Work out the finished part from the listing and answer in its coordinate system (mm). A direction names the side the tool comes from. Give positions to 0.01 mm unless a question says otherwise; leave off trailing zeros. Order: outer loops, then holes, each group sorted by start corner. A loop starts at its lowest first (then second) coordinate and runs counter-clockwise, first axis right, second up.
```python
from build123d import *

# Parameters (mm, degrees)
F0_R            = 125
F1_DEPTH        = 1000
F6_DEPTH        = 25
F6_COPIES_COUNT = 6


# Not quite as in the source:
# - a fillet or chamfer that OpenCascade refuses, or shapes differently, is made with other operations: its cross-section is extruded or revolved along the edge and cut away or added
# - a pattern or mirror of a feature is missing from the dataset's text; its kind, count and spacing are read off the source's solid


with BuildPart() as f1:
    # F0 (on Top) → F1 (new body)
    with BuildSketch(Plane.XY):
        Circle(F0_R)
    extrude(amount=F1_DEPTH)

    # F2 (on Front) → F3 (revolve)
    with BuildSketch(Plane.XZ):
        Polygon((-124.5536804199, 997.6518154144), (0, 998.6120462418), (0, 1213.404417038), align=None)
    revolve(axis=Axis((0, 0, 1106.0082316399), (0, 0, 1)))

    # F4: fillet of radius 5 on 1 edges, made by hand

    # F4_s1 → F4_t2 (revolve, cut)
    with BuildSketch(Plane.XZ):
        with BuildLine():
            ThreePointArc((125, 996.1565242927), (124.5271615516, 998.2789776575), (123.1980766857, 1000))
            Line((123.1980766857, 1000), (125, 1000))
            Line((125, 1000), (125, 996.1565242927))
        make_face()
    revolve(axis=Axis((0, 0, 1000), (0, 0, 1)), mode=Mode.SUBTRACT)

    # F5 (on Front) → F6 (join)
    with BuildSketch(Plane.XZ):
        Polygon((0, 300), (0, 0), (250, 0), align=None)
    f6 = extrude(amount=F6_DEPTH)

    # F6_copies: F6 ×6 about axis
    f6_copies_axis = Axis((0, 0, 0), (0, 0, 1))
    for i in range(1, F6_COPIES_COUNT):
        add(f6.rotate(f6_copies_axis, i * 360 / F6_COPIES_COUNT))


solid = f1.part
```
1. Which of the six approach directions +Z, -Z, +X, -X, +Y, -Y give full straight-line access (tool end or side, diameter ignored) to faces 1 (the face through (56.85, -148.47, 43.58)), 2 (the face through (79.424, -137.566, 42.717)), 3 (the face through (-56.85, 148.47, 43.58)), 4 (the face through (-100.153, -123.471, 43.58)), 5 (the face through (-124.88, 5.5, 491.11))?
Findings below:
face 1: +Z, -Z, -Y
face 2: +Z, -Z, +X
face 3: +Z, -Z, +Y
face 4: +Z, -Z, -X
face 5: +Z
2. The part is cut by section C-C (x = 207.5). Write down the section's boundary in (y, z), then the cut area to 4 significant figures.
Findings below:
outline: (-25, 0) - (0, 0) - (0, 51) - (-25, 51) - close
area: 1,275 mm2
3. The mould has two halves that part along X. Classify faces 6 (the face through (-79.424, -137.566, 42.717)), 7 (the face through (187.13, -12.325, 75.444)), 8 (the face through (-104.24, -155.9, 75.44)): pulls with the +X half, pulls with the -X half, needs draft (parallel to the pull), parting line crosses it, or undercut.
Findings below:
face 6: undercut
face 7: pulls with the +X half
face 8: pulls with the -X half
4. Given P1, Ø10, axis at x = -110, z = 275, coming from the -Y side; P2, Ø12, axis at x = 56, y = -46.5, coming from the -Z side; P3, Ø10, axis at x = -53, z = 622, coming from the -Y side; P4, Ø1, axis at y = -35, z = 1061.5, coming from the -X side, each flat-ended and moving along its own axis, determine where each tip first touches the part or whether it passes through.
Findings below:
P1: stops at y = -67.82
P2: stops at z = 0
P3: stops at y = -115.42
P4: stops at x = -80.79
5. The part is cut by section A-A (y = 169). Write down the section's boundary in (x, z).
Findings below:
outline: (-97.57, 0) - (-68.7, 0) - (-68.7, 83.15) - (-97.57, 65.83) - close; (97.57, 0) - (126.44, 0) - (126.44, 48.51) - (97.57, 65.83) - close
6. Straight lines are drawn through the part: probe 1 along X at (y, z) = (-6, 374.5); probe 2 along X at (y, z) = (-24.5, 182.5); probe 3 along Z at (x, y) = (54, -77). For each, find the intervals that lie inside material, in ascending order.
Findings below:
probe 1: x = -124.86 to 124.86
probe 2: x = -122.58 to 122.58
probe 3: z = 0 to 1050.49
7. The part is cut by section D-D (z = 1094.5). Write down the section's boundary in (x, y).
Findings below:
outline: circle Ø137.29 at (0, 0)
8. The part is cut by section B-B (z = 791). Write down the section's boundary in (x, y), then the cut area to 3 significant figures.
Findings below:
outline: circle Ø250 at (0, 0)
area: 49,100 mm2
